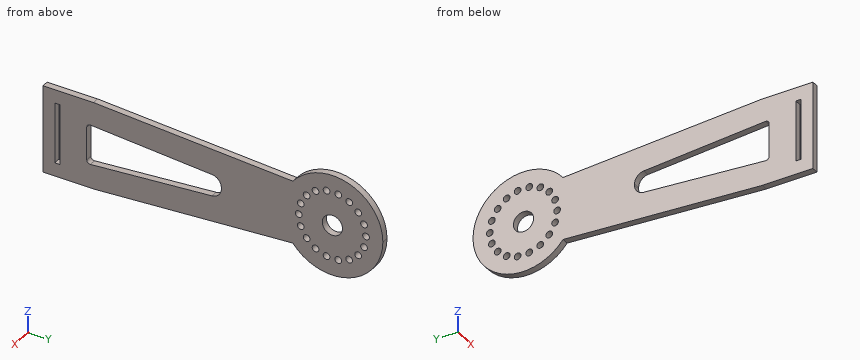
```python
from build123d import *

# Parameters (mm, degrees)
RESSALTO_EXTRUS_O1_DEPTH = 2
ESBO_O2_R                = 3
ESBO_O2_R_2              = 1
CORTE_EXTRUS_O1_DEPTH    = 2
PADR_OCIRCULAR1_COUNT    = 18
ESBO_O3_W                = 18
ESBO_O3_H                = 1.561418551
CORTE_EXTRUS_O2_DEPTH    = 2


with BuildPart() as part:
    # Esboço1 → Ressalto-extrusão1 (new body)
    with BuildSketch(Plane(origin=(0, 0, 0), x_dir=(0, 0, -1), z_dir=(1, 0, 0))):
        with BuildLine():
            Line((-13, -71), (-13, -86))
            Line((-13, -86), (0, -86))
            Line((0, -86), (0, 15))
            ThreePointArc((0, 15), (-14.165790836, 4.932582487), (-9.316524238, -11.755950669))
            add(Edge.make_bspline(
                [(-9.316524238, -11.755950669), (-13, -71)],
                knots=[0, 0, 1, 1], degree=1))
        make_face()
    ressalto_extrus_o1 = extrude(amount=RESSALTO_EXTRUS_O1_DEPTH)

    # Espelhar1: Ressalto-extrusão1 across plane
    add(ressalto_extrus_o1.mirror(Plane(origin=(2, 15, 0), x_dir=(1, 0, 0), z_dir=(0, 0, 1))))

    # Esboço2 → Corte-extrusão1 (cut)
    with BuildSketch(Plane(origin=(2, 0, 0), x_dir=(0, 0, -1), z_dir=(1, 0, 0))):
        Circle(ESBO_O2_R)
        with Locations((0, -10)):
            Circle(ESBO_O2_R_2)
    corte_extrus_o1 = extrude(amount=-CORTE_EXTRUS_O1_DEPTH, mode=Mode.SUBTRACT)

    # PadrãoCircular1: Corte-extrusão1 ×18 about axis
    padr_ocircular1_axis = Axis((0, 0, 0), (1, 0, 0))
    for i in range(1, PADR_OCIRCULAR1_COUNT):
        add(corte_extrus_o1.rotate(padr_ocircular1_axis, i * 360 / PADR_OCIRCULAR1_COUNT), mode=Mode.SUBTRACT)

    # Esboço3 → Corte-extrusão2 (cut)
    with BuildSketch(Plane(origin=(2, 0, 0), x_dir=(0, 0, -1), z_dir=(1, 0, 0))):
        with BuildLine():
            Line((-4.922191444, -73), (4.922191444, -73))
            ThreePointArc((4.922191444, -73), (5.655263728, -72.680150738), (5.919390754, -71.925210052))
            Line((5.919390754, -71.925210052), (3.208172262, -35.775630155))
            ThreePointArc((3.208172262, -35.775630155), (2.257026545, -33.800783147), (0.216574332, -33))
            Line((0.216574332, -33), (-0.216574332, -33))
            ThreePointArc((-0.216574332, -33), (-2.257026545, -33.800783147), (-3.208172262, -35.775630155))
            Line((-3.208172262, -35.775630155), (-5.919390754, -71.925210052))
            ThreePointArc((-5.919390754, -71.925210052), (-5.655263728, -72.680150738), (-4.922191444, -73))
        make_face()
        with Locations((0, -81.719290725)):
            Rectangle(ESBO_O3_W, ESBO_O3_H)
    extrude(amount=-CORTE_EXTRUS_O2_DEPTH, mode=Mode.SUBTRACT)


solid = part.part
```
Source: CAD feature listing. Evaluate the final solid. Frame: model axes, mm. Coordinates: 2 decimals unless noted, no trailing zeros. Loops run counter-clockwise (first coordinate to the right, second up) from the corner with the lowest first, then second, coordinate; pieces in that order, holes last. Notation, with made-up numbers: M 57,27.5 L 73,27.5 A32 cw 73,63.5 Z; hole C 7,1 d5. An arc over 180 degrees is marked long. Put each result on its own line as item: value. Start each with the question number.
1) Contact query for flat-ended pins moving along their axis: pin 1 Ø2.5 at (y, z) = (1.74, 9.85) entering from +X; pin 2 Ø1 at (x, y) = (1, -78.5) entering from -Z; pin 3 Ø0.6 at (x, z) = (1, 4.5) entering from +Y. Output: stop coordinate, or through.
2) Cut plane A-A on y = 5. Return the cut outline in (x, z).
3) Ray query, L1, parallel to Y at x = 1, z = -1.5; L2, parallel to Z at x = 0.2, y = 10; L3, parallel to Y at x = 1.7, z = -8. Return the intervals inside material, ascending. Write a range as from..to.
The answers:
1. pin 1: stops at x = 2
1. pin 2: stops at z = -13
1. pin 3: stops at y = 14.4
2. outline: M 0,-14.14 L 2,-14.14 L 2,-9.66 L 0,-9.66 Z; M 0,-7.66 L 2,-7.66 L 2,7.66 L 0,7.66 Z; M 0,9.66 L 2,9.66 L 2,14.14 L 0,14.14 Z
3. L1: y = -86..-82.5, -80.94..-73, -33.29..-2.6, 2.6..14.92
3. L2: z = -11.18..-4.22, -2.62..-1, 1..2.62, 4.22..11.18
3. L3: y = -86..-82.5, -80.94..-5.75, -4.25..4.25, 5.75..12.69
